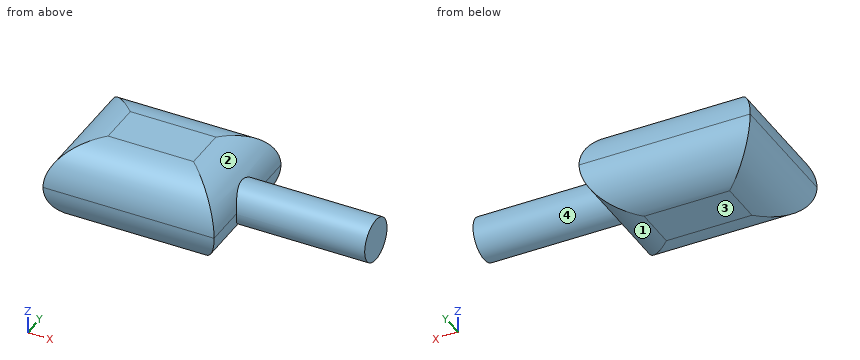
```python
from build123d import *

# Parameters (mm, degrees)
F0_W     = 20
F0_H     = 15
F1_DEPTH = 5
F2_R     = 4.99999
F3_R     = 2.5
F4_DEPTH = 25


# Not quite as in the source:
# - a fillet or chamfer is up to 0.001 mm smaller than in the source, because OpenCascade refuses the exact size


with BuildPart() as f1:
    # F0 (on Top) → F1 (new body, symmetric)
    with BuildSketch(Plane.XY):
        Rectangle(F0_W, F0_H)
    extrude(amount=F1_DEPTH, both=True)

    # F2 (radius 5 in the source; OpenCascade refuses exactly that, so slightly less here)
    f2_edges = [f1.edges().sort_by_distance(p)[0] for p in [
        (0, 7.5, 5),
        (-10, 0, 5),
        (0, -7.5, 5),
        (10, 0, 5),
        (0, -7.5, -5),
        (10, 0, -5),
        (0, 7.5, -5),
        (-10, 0, -5),
    ]]
    fillet(f2_edges, radius=F2_R)

    # F3 (on Right) → F4 (join)
    with BuildSketch(Plane.YZ):
        Circle(F3_R)
    extrude(amount=F4_DEPTH)


solid = f1.part
```
Part model, mm, in its own coordinate system. Face numbers are marked on the shaded views. A direction names the side the tool comes from. Round coordinates to 2 decimals unless told otherwise and drop trailing zeros. Write each loop counter-clockwise with the first axis right and the second up, starting at its lowest first coordinate (ties: lowest second). Pieces come first, ordered by that corner, then holes. Notation, with made-up numbers: (41.25, 66) -> (94.25, 66) arc R13 cw to (94.25, 78) -> close; hole circle Ø10 at (80.25, 60). An arc over 180 degrees is marked (long way). Return JSON: item names as keys, results as strings. Group by question number.
Q1. Saw through at C-C on z = 3. Write the cut outline in (x, y), plus the area to 3 significant figures.
Q2. Which spindle directions (+Z, -Z, +X, -X, +Y, -Y) get a long thin tool onto all of the face, cutting with end or side? Do the marked faces 1, 2, 3 and 4. Say none if no direction does.
Q3. Pin check, flat tips, straight feed: pin 1 (2 mm diameter, centred on y = 2, z = 4, fed in from -X); pin 2 (6 mm diameter, centred on y = -3, z = -4, fed in from -X); pin 3 (5 mm diameter, centred on x = 21.5, z = -2.5, fed in from +Y). Stop position of each tip, or through.
Q4. Probe L1, parallel to Y at x = 5, z = 0.25; L2, parallel to X at y = 3.25, z = 2.5; L3, parallel to Z at x = 4, y = 5. List the from-to ranges inside material, lowest first. Write a range as [from, to].
Answer:
{
 "1": {"outline": "(-9, -6.5) -> (9, -6.5) -> (9, 6.5) -> (-9, 6.5) -> close", "area": "234 mm2"},
 "2": {"face 1": "-Z, +X", "face 2": "+Z, +X", "face 3": "-Z, +X, -X, +Y, -Y", "face 4": "+X"},
 "3": {"pin 1": "x = -9", "pin 2": "x = -9.9", "pin 3": "y = 2.5"},
 "4": {"L1": "[-7.49, 7.49]", "L2": "[-9.33, 9.33]", "L3": "[-4.33, 4.33]"}
}
